Autodesk Inventor part; units mm, degrees
ref_plane "YZ Plane" through (0, 0, 0) normal (1, 0, 0) x (0, 1, 0)
ref_plane "XZ Plane" through (0, 0, 0) normal (0, 1, 0) x (-1, 0, 0)
ref_plane "XY Plane" through (0, 0, 0) normal (0, 0, 1) x (1, 0, 0)
sketch "スケッチ1" plane through (0, 0, 0) normal (1, 0, 0) x (0, 1, 0)
  line L0 (12.1, 0) -> (12.1, 5)
  line L1 (12.1, 5) -> (10.1, 5)
  line L2 (10.1, 5) -> (10.1, 22)
  line L3 (23.9, 20) -> (37.5, 20)
  line L4 (37.5, 20) -> (37.5, 0)
  line L5 (37.5, 0) -> (12.1, 0)
  line L6 (0, -4.4) -> (0, 26.4)
  line L7 (23.9, 20) -> (23.9, 22)
  line L8 (23.9, 22) -> (10.1, 22)
  point P0 (0, 0)
  dimension "d0" = 12.1
  dimension "d1" = 37.5
  dimension "d2" = 2
  dimension "d3" = 5
  dimension "d5" = 20
  dimension "d28" = 2
  dimension "d29" = 23.9
revolve "回転1" add sketch "スケッチ1" angle 360 about axis through (0, 0, -10) along (0, 0, 1)
chamfer "面取り1" distance 0.5 angle 45 1 edges at (0, -12.1, 0)
sketch "スケッチ2" plane through (0, 0, 20) normal (0, 0, 1) x (1, 0, 0)
  circle A0 centre (0, 0) radius 32
  point P0 (0, 32)
  point P1 (-27.7128, 16)
  point P2 (-27.7128, -16)
  point P3 (0, -32)
  point P4 (27.7128, -16)
  point P5 (27.7128, 16)
  dimension "d10" = 64
  dimension "d13" = 360
hole "穴1" at (0, 32, 20) at (-27.7128, 16, 20) at (-27.7128, -16, 20) at (0, -32, 20) at (27.7128, -16, 20) at (27.7128, 16, 20) direction (0, 0, -1) diameter 4.3 end through all
chamfer "面取り2" distance 1 angle 45 2 edges at (0, -37.5, 0) (0, -37.5, 20)
chamfer "面取り3" distance 0.5 angle 45 1 edges at (0, -23.9, 22)
properties part number "unit-base2" material "ABS プラスチック"
Can you work these out from the model? Positions are in its coordinate system, mm. A direction names the side the tool comes from. Coordinates: 2 decimals unless noted, no trailing zeros. Order: outer loops, then holes, each group sorted by start corner. A loop starts at its lowest first (then second) coordinate and runs counter-clockwise, first axis right, second up.
1. I need wall thicknesses on line 1 (Y direction, x = 0, z = 9.75); line 2 (Y direction, x = -1.5, z = 10.5); line 3 (X direction, y = 0, z = 10). Which ranges of each line are inside material? Lowest first, please.
2. I'm going to push flat-ended pins straight in: pin 1 (8 mm diameter, centred on x = 19.5, z = 12, fed in from +Y); pin 2 (5 mm diameter, centred on y = -8.5, z = 16, fed in from +X); pin 3 (4 mm diameter, centred on y = 8.5, z = 6.5, fed in from +X). Where does each tip first touch, or does it pass through?
3. If we section it at B-B (x = 0): Give the number of separate pieces and of enclosed holes in the cut face, then the cut area to 3 significant figures.
4. For faces 4 (the face through (10, -3, 5)), 5 (the face through (-20.15, 12.85, 20.76)), 6 (the face through (-3.034, 9.634, 13.619)), which set-ups out of +Z, -Z, +X, -X, +Y, -Y let a thin tool reach every point of the face, with its end or its side?
5. If we section it at A-A (y = 0): Please give me the cut outline in (x, z).
6. If we section it at C-C (z = 8.25): Please give me the cut outline in (x, y).
7. Thinking about a two-plate mould opening in X: for faces 1 (the face through (4.63, 11.18, 2.78)), 2 (the face through (37.18, -4.88, 9.87)), 3 (the face through (8, 24, 20)), which applies, +X half, -X half, draft (parallel to the pull), parting line (faces both ways), or undercut?
Entries:
1. line 1: y = -37.5 to -34.15, -29.85 to -10.1, 10.1 to 29.85, 34.15 to 37.5
1. line 2: y = -37.47 to -33.54, -30.46 to -9.99, 9.99 to 30.46, 33.54 to 37.47
1. line 3: x = -37.5 to -10.1, 10.1 to 37.5
2. pin 1: stops at y = 34.15
2. pin 2: stops at x = 37.02
2. pin 3: stops at x = 36.93
3. separate pieces: 4
3. enclosed holes: 0
3. area: 957 mm2
4. face 4: -Z
4. face 5: +Z
4. face 6: +Z, -Z
5. outline: (-37.5, 1) - (-36.5, 0) - (-12.6, 0) - (-12.1, 0.5) - (-12.1, 5) - (-10.1, 5) - (-10.1, 22) - (-23.4, 22) - (-23.9, 21.5) - (-23.9, 20) - (-36.5, 20) - (-37.5, 19) - close; (10.1, 5) - (12.1, 5) - (12.1, 0.5) - (12.6, 0) - (36.5, 0) - (37.5, 1) - (37.5, 19) - (36.5, 20) - (23.9, 20) - (23.9, 21.5) - (23.4, 22) - (10.1, 22) - close
6. outline: circle Ø75 at (0, 0); hole circle Ø4.3 at (-27.71, -16); hole circle Ø4.3 at (-27.71, 16); hole circle Ø20.2 at (0, 0); hole circle Ø4.3 at (0, -32); hole circle Ø4.3 at (0, 32); hole circle Ø4.3 at (27.71, -16); hole circle Ø4.3 at (27.71, 16)
7. face 1: undercut
7. face 2: parting line
7. face 3: draft
